Design review of the part built by this model. Coordinates are the model's own, in mm. Face numbers are marked on the shaded views. Coordinates: 2 decimals unless noted, no trailing zeros. Loops run counter-clockwise (first coordinate to the right, second up) from the corner with the lowest first, then second, coordinate; pieces in that order, holes last. Notation, with made-up numbers: (3, 34) -> (50, 34) arc R29 ccw to (50, 55) -> close; hole circle Ø6 at (-35.75, -28.75). An arc over 180 degrees is marked (long way). Use a Markdown table: item, result. Add a question column.
Q1. Clearance check with flat-ended pins moving along their axes: pin 1 Ø3 at (y, z) = (7.5, -88) entering from -X; pin 2 Ø1.5 at (y, z) = (7.5, 57.5) entering from -X; pin 3 Ø6 at (x, y) = (-16.5, 8) entering from +Z; pin 4 Ø2 at (y, z) = (7.5, 88) entering from +X. State where each tip first meets the part, or that it passes through.
Q2. Take a section at D-D on x = -68. Write out the cut boundary in (y, z).
Q3. Draft analysis for pull direction Z (two halves, no side actions). For the marked faces 1, 2 and 3, state which applies: pulls with the +Z half, pulls with the -Z half, needs draft (parallel to the pull), parting line crosses it, or undercut.
Q4. For probe 1 along Y at (x, z) = (-2, 88); probe 2 along Z at (x, y) = (-2.5, 7.5); probe 3 along Z at (x, y) = (-6, 7.5), list the stretches that pass through material, from the lowest coordinate up.
Q5. Take a section at C-C on z = 0. Write out the cut boundary in (x, y), plus the area to 3 significant figures.
Q6. Take a section at B-B on x = -50. Write out the cut boundary in (y, z).
Q7. Take a section at A-A on x = -24.5. Write out the cut boundary in (y, z), plus the area to 3 significant figures.
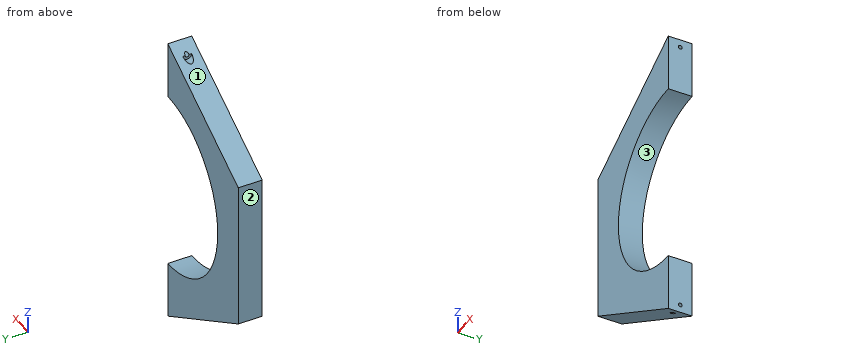
Autodesk Inventor part; units mm, degrees
ref_plane "作業平面3" through (-8.6603, 7.5, 88) normal (0, 0, -1) x (-1, 0, 0)
ref_plane "作業平面4" through (-13.4603, 7.5, 88) normal (-1, 0, 0) x (0, 0, 1)
ref_plane "作業平面5" through (0, 15, 0) normal (0, 0, 1) x (1, 0, 0)
sketch "スケッチ1" plane through (0, 0, 0) normal (0, 1, 0) x (-1, 0, 0)
  arc A0 (0, -57) -> (0, 57) centre (0, 0) ccw
  line L0 (0, 0) -> (80.5404, 46.5) construction
  line L1 (0, 0) -> (0, 93) construction
  line L2 (0, 93) -> (80.5404, 46.5)
  line L3 (80.5404, 46.5) -> (80.5404, 0)
  line L4 (80.5404, 0) -> (57, 0)
  line L5 (0, 0) -> (0, -93) construction
  line L6 (0, -93) -> (80.5404, -46.5)
  line L7 (80.5404, -46.5) -> (80.5404, 0)
  line L8 (0, -93) -> (0, -57)
  line L9 (0, 93) -> (0, 57)
  dimension "d0" = 57
extrude "押し出し1" add sketch "スケッチ1" along normal blind 15
sketch "スケッチ2" plane through (0, 0, 93) normal (1, 0, 0) x (0, 0, -1)
  line L0 (36, 0) -> (36, 15)
  line L1 (36, 15) -> (5, 15)
  line L2 (46.5, 15) -> (0, 15)
  line L3 (5, 15) -> (5, 7.5)
  line L4 (93, 0) -> (93, 15)
  line L5 (139.5, 15) -> (46.5, 15)
  line L6 (181, 15) -> (181, 7.5)
  dimension "d5" = 31
  dimension "d6" = 7.5
hole "穴1" at (0, 7.5, 88) direction (-1, 0, 0) diameter 2.459 end through all
sketch "スケッチ3" plane through (0, 0, 93) normal (-0.5, 0, 0.866) x (0.866, 0, 0.5)
  ellipse E0 centre (-10, 7.5) end of major axis (-12.459, 7.5) minor radius 1.2295
  point P0 (-46.5, 0)
  point P1 (-7.541, 7.5)
sketch "スケッチ5" plane through (0, 0, 93) normal (-0.5, 0, 0.866) x (0.866, 0, 0.5)
  ellipse E0 centre (-10, 7.5) end of major axis (-12.459, 7.5) minor radius 1.2295
  point P0 (-46.5, 0)
  point P1 (-12.459, 7.5)
ref_plane "作業平面3" through (-8.6603, 7.5, 88) normal (0, 0, -1) x (-1, 0, 0)
sketch "スケッチ7" plane through (-8.6603, 7.5, 88) normal (0, 0, -1) x (-1, 0, 0)
  line L0 (0, 0) -> (4.8, 0)
  point P0 (-8.6603, -7.5)
  dimension "d21" = 4.8
ref_plane "作業平面4" through (-13.4603, 7.5, 88) normal (-1, 0, 0) x (0, 0, 1)
sketch "スケッチ8" plane through (-13.4603, 7.5, 88) normal (-1, 0, 0) x (0, 0, 1)
  point P0 (-88, -7.5)
  point P1 (0, 0)
hole "穴3" at (-13.4603, 7.5, 88) direction (1, 0, 0) diameter 2.459 end through all counterbore diameter 5.5 counterbore depth 5
sketch "スケッチ9" plane through (0, 15, 0) normal (0, 1, 0) x (1, 0, 0)
  point P0 (0, 0)
  point P1 (0, 0)
ref_plane "作業平面5" through (0, 15, 0) normal (0, 0, 1) x (1, 0, 0)
hole "穴4" at (0, 7.5, -88) direction (-1, 0, 0) diameter 2.459 end through all
properties part number "nowtrying_up"
Answer list:
| question | item | result |
|---|---|---|
| 1 | pin 1 | x = -11.26 |
| 1 | pin 2 | x = -62.79 |
| 1 | pin 3 | z = 85.21 |
| 1 | pin 4 | through |
| 2 | outline | (0, -53.74) -> (15, -53.74) -> (15, 53.74) -> (0, 53.74) -> close |
| 3 | face 1 | pulls with the +Z half |
| 3 | face 2 | needs draft |
| 3 | face 3 | undercut |
| 4 | probe 1 | 0 to 6.27, 8.73 to 15 |
| 4 | probe 2 | -91.56 to -89.23, -86.77 to -56.95, 56.95 to 86.77, 89.23 to 91.56 |
| 4 | probe 3 | -89.54 to -89.23, -86.77 to -56.68, 56.68 to 86.77, 89.23 to 89.54 |
| 5 | outline | (-80.54, 0) -> (-57, 0) -> (-57, 15) -> (-80.54, 15) -> close |
| 5 | area | 353 mm² |
| 6 | outline | (0, -64.13) -> (15, -64.13) -> (15, -27.37) -> (0, -27.37) -> close; (0, 27.37) -> (15, 27.37) -> (15, 64.13) -> (0, 64.13) -> close |
| 7 | outline | (0, -78.85) -> (15, -78.85) -> (15, -51.47) -> (0, -51.47) -> close; (0, 51.47) -> (15, 51.47) -> (15, 78.85) -> (0, 78.85) -> close |
| 7 | area | 822 mm² |
